Input: part model. Units: mm. Frame: model coordinates. Face numbers are marked on the shaded views. A direction names the side the tool comes from. Coordinates: 2 decimals unless noted, no trailing zeros. Loops run counter-clockwise (first coordinate to the right, second up) from the corner with the lowest first, then second, coordinate; pieces in that order, holes last.
(1) Set-up query: the marked faces 1 and 2. Return all of +Z, -Z, +X, -X, +Y, -Y with unobstructed straight access to the full face (end or side cutting, diameter ignored); none if empty.
(2) Line query: L1, parallel to Z at x = 34.5, y = 0 (3 decimals); L2, parallel to Y at x = 25, z = 0.25. Output: solid intervals per line, ascending.
(3) Section A-A, the plane x = -56. Return loops of the section in (y, z).
(4) Contact query for flat-ended pins moving along their axis: P1, Ø10, axis at x = 17, z = 8, coming from the +Y side; P2, Ø8, axis at x = -3.5, z = 9.5, coming from the -Y side; P3, Ø2, axis at x = -7, z = -10, coming from the -Y side. Output: stop coordinate, or through.
```python
from build123d import *

# Parameters (mm, degrees)
F3_D     = 6.9088
F3_DEPTH = 28.575
F3_TIP   = 2.0756129224
F4_R     = 9.525
F5_DEPTH = 2.38125
F6_R     = 0.508
F7_SIZE  = 0.762


with BuildPart() as f1:
    # F0 (on Front) → F1 (revolve)
    with BuildSketch(Plane.XZ):
        Polygon((-101.6, 12.7), (-101.6, 0), (47.625, 0), (47.625, 9.525), (0, 9.525), (0, 12.7), align=None)
    revolve(axis=Axis((-26.9875, 0, 0), (1, 0, 0)))

    # F3
    with Locations(Plane.YZ.offset(47.625)):
        with Locations((0, 0)):
            Hole(F3_D / 2, depth=F3_DEPTH)
            with Locations((0, 0, -(F3_DEPTH + F3_TIP / 2))):  # 118° drill point
                Cone(0, F3_D / 2, F3_TIP, mode=Mode.SUBTRACT)

    # F4 (on Front) → F5 (cut, symmetric)
    with BuildSketch(Plane.XZ):
        with Locations((11.1125, 12.954)):
            Circle(F4_R)
    extrude(amount=F5_DEPTH, both=True, mode=Mode.SUBTRACT)

    # F6
    f6_edges = [f1.edges().sort_by_distance(p)[0] for p in [
        (0, 0, -9.525),
    ]]
    fillet(f6_edges, radius=F6_R)

    # F7
    f7_edges = [f1.edges().sort_by_distance(p)[0] for p in [
        (-101.6, 0, -12.7),
        (47.625, 0, -9.525),
    ]]
    chamfer(f7_edges, length=F7_SIZE)


solid = f1.part
```
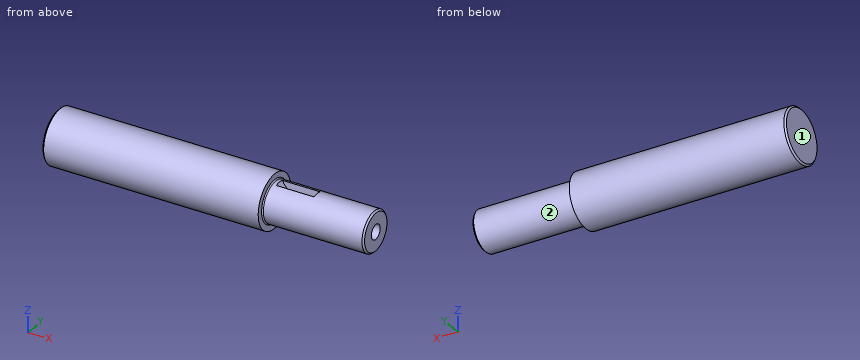
Report:
1. face 1: +Z, -Z, -X, +Y, -Y
1. face 2: +X
2. L1: z = -9.525 to -3.454, 3.454 to 9.525
2. L2: y = -9.52 to -3.45, 3.45 to 9.52
3. outline: circle Ø25.4 at (0, 0)
4. P1: stops at y = 9.04
4. P2: stops at y = -11.45
4. P3: stops at y = -8.96
